Can you work these out from the model? Positions are in its coordinate system, mm. Face numbers are marked on the shaded views. A direction names the side the tool comes from. Round coordinates to 2 decimals unless told otherwise and drop trailing zeros. Write each loop counter-clockwise with the first axis right and the second up, starting at its lowest first coordinate (ties: lowest second). Pieces come first, ordered by that corner, then holes. Notation, with made-up numbers: (83, 85) - (100, 85) arc R28 cw to (100, 111) - close; hole circle Ø5 at (42, -29.5). An arc over 180 degrees is marked (long way). One line per item, written item: value. Start each with the question number.
(1) I'm going to push flat-ended pins straight in: pin 1 Ø5 at (x, y) = (-11, 5.5) entering from -Z; pin 2 Ø14 at (y, z) = (-3, 5.5) entering from -X; pin 3 Ø4 at (x, z) = (-13.5, -3) entering from +Y. Where does each tip first touch, or does it pass through?
(2) I want a section at D-D on x = -9. List the corners of the cut face in (y, z) for me, plus the area to 3 significant figures.
(3) I want a section at C-C on x = 0. List the corners of the cut face in (y, z) for me.
(4) Thinking about a two-plate mould opening in X: for the marked faces 4, 5 and 6, which applies, +X half, -X half, draft (parallel to the pull), parting line (faces both ways), or undercut?
(5) If I drill on L1, parallel to Y at x = 0, z = 2.75; L2, parallel to Z at x = -8, y = -17; L3, parallel to Z at x = -12, y = 1, over which ranges is the centre line in solid material (lowest first)? Write a range as from..to.
(6) I want a section at A-A on z = -23. List the corners of the cut face in (x, y) for me, plus the area to 3 significant figures.
(7) I want a section at B-B on y = 0. List the corners of the cut face in (x, z) for me, plus the area to 3 significant figures.
(8) On a 3-axis mill with a long thin cutter (end or side, diameter ignored), from which of +Z, -Z, +X, -X, +Y, -Y can I reach the whole of each face in a straight line? I mean the marked faces 1, 2 and 3. Say none if no direction works.
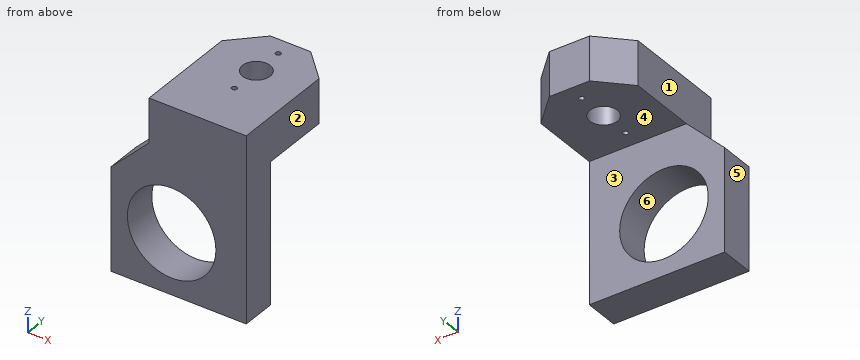
from build123d import *

# Parameters (mm, degrees)
SKETCH1_R           = 4
SKETCH1_R_2         = 0.75
BOSS_EXTRUDE1_DEPTH = 12.7
SKETCH2_R           = 12.75
BOSS_EXTRUDE2_DEPTH = 10


with BuildPart() as part:
    # Sketch1 → Boss-Extrude1 (new body)
    with BuildSketch(Plane.XY):
        Polygon((-5.798989873, 14), (5.798989873, 14), (14, 5.798989873), (14, -5.798989873), (14, -14), (5.798989873, -14), (-5.798989873, -14), (-14, -14), (-14, -5.798989873), (-14, 5.798989873), align=None)
        Circle(SKETCH1_R, mode=Mode.SUBTRACT)
        with Locations((0, 9)):
            Circle(SKETCH1_R_2, mode=Mode.SUBTRACT)
        with Locations((0, -9)):
            Circle(SKETCH1_R_2, mode=Mode.SUBTRACT)
    extrude(amount=BOSS_EXTRUDE1_DEPTH)

    # Sketch2 → Boss-Extrude2 (add)
    with BuildSketch(Plane.XZ.offset(14)):
        Polygon((14, 12.7), (-14, 12.7), (-14, 0), (-25, -11), (-25, -40.5), (14, -40.5), align=None)
        with Locations((-7.5, -23)):
            Circle(SKETCH2_R, mode=Mode.SUBTRACT)
    extrude(amount=BOSS_EXTRUDE2_DEPTH)


solid = part.part
Established:
1. pin 1: z = 0
1. pin 2: x = -14
1. pin 3: y = -14
2. outline: (-24, -40.5) - (-14, -40.5) - (-14, -35.66) - (-24, -35.66) - close; (-24, -10.34) - (-14, -10.34) - (-14, 0) - (10.8, 0) - (10.8, 12.7) - (-24, 12.7) - close
2. area: 594 mm2
3. outline: (-24, -40.5) - (-14, -40.5) - (-14, -33.31) - (-24, -33.31) - close; (-24, -12.69) - (-14, -12.69) - (-14, 0) - (-9.75, 0) - (-9.75, 12.7) - (-24, 12.7) - close; (-8.25, 0) - (-4, 0) - (-4, 12.7) - (-8.25, 12.7) - close; (4, 0) - (8.25, 0) - (8.25, 12.7) - (4, 12.7) - close; (9.75, 0) - (14, 0) - (14, 12.7) - (9.75, 12.7) - close
4. face 4: draft
4. face 5: -X half
4. face 6: undercut
5. L1: -24..-9.75, -8.25..-4, 4..8.25, 9.75..14
5. L2: -40.5..-35.74, -10.26..12.7
5. L3: 0..12.7
6. outline: (-25, -24) - (-20.25, -24) - (-20.25, -14) - (-25, -14) - close; (5.25, -24) - (14, -24) - (14, -14) - (5.25, -14) - close
6. area: 135 mm2
7. outline: (-14, 0) - (-4, 0) - (-4, 12.7) - (-14, 12.7) - close; (4, 0) - (14, 0) - (14, 12.7) - (4, 12.7) - close
7. area: 254 mm2
8. face 1: +Z, -X, +Y, -Y
8. face 2: +Z, -Z, +X, +Y, -Y
8. face 3: -Z, +X, -X, +Y
